Input: part model. Units: mm. Frame: model coordinates. Face numbers are marked on the shaded views. A direction names the side the tool comes from. Give positions to 0.01 mm unless a question says otherwise; leave off trailing zeros. Loops run counter-clockwise (first coordinate to the right, second up) from the corner with the lowest first, then second, coordinate; pieces in that order, holes last. Notation, with made-up numbers: M 54.5,-30 L 98.5,-30 A28 cw 98.5,1 Z; hole C 54,9.5 d7. An arc over 180 degrees is marked long. One line per item, written item: value. Start each with the question number.
(1) Ray query, line 1 along X through (y, z) = (1.4, 15); line 2 along Y through (x, z) = (0.75, 2); line 3 along Z through (x, y) = (-5, -0.2). Return the intervals inside material, ascending. Write a range as from..to.
(2) Section D-D on x = -1.25. Output: boundary loops of the cut face in (y, z), plus the area to 3 significant figures.
(3) Pin query (flat end, axial travel): P1, Ø0.5, axis at y = 1.5, z = 14.5, coming from the +X side; P2, Ø0.5, axis at x = -5.5, z = 7.5, coming from the -Y side; P3, Ø2, axis at y = -0.5, z = -1.5, coming from the -X side. Return the tip coordinate at first contact, or that it passes through.
(4) Access query for the marked faces 1 and 2. Directions: +Z, -Z, +X, -X, +Y, -Y. A direction counts if a zero-diameter tool reaches every point of the face in a straight line with its end or side. Return the directions, or none.
(5) Section C-C on x = 5.25. Output: boundary loops of the cut face in (y, z).
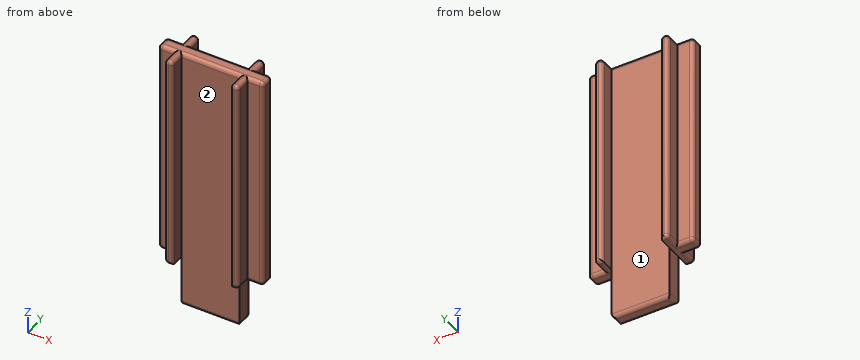
```python
from build123d import *

# Parameters (mm, degrees)
AUFSATZ_LINEAR_AUSTRAGEN1_DEPTH = 28
SKIZZE2_W                       = 7.5
SKIZZE2_H                       = 1.8
AUFSATZ_LINEAR_AUSTRAGEN2_DEPTH = 6.63
VERRUNDUNG1_R                   = 0.5


with BuildPart() as part:
    # Skizze1 → Aufsatz-Linear austragen1 (new body)
    with BuildSketch(Plane.XY):
        Polygon((-4.75, 0.9), (-6.8, 0.9), (-6.8, -0.9), (-4.75, -0.9), (-4.75, -2.9), (-3.75, -2.9), (-3.75, -0.9), (3.75, -0.9), (3.75, -2.9), (4.75, -2.9), (4.75, -0.9), (6.8, -0.9), (6.8, 0.9), (4.75, 0.9), (4.75, 2.9), (3.75, 2.9), (3.75, 0.9), (-3.75, 0.9), (-3.75, 2.9), (-4.75, 2.9), align=None)
    extrude(amount=AUFSATZ_LINEAR_AUSTRAGEN1_DEPTH)

    # Skizze2 → Aufsatz-Linear austragen2 (add)
    with BuildSketch(Plane(origin=(0, 0, 0), x_dir=(-1, 0, 0), z_dir=(0, 0, -1))):
        Rectangle(SKIZZE2_W, SKIZZE2_H)
    extrude(amount=AUFSATZ_LINEAR_AUSTRAGEN2_DEPTH)

    # Verrundung1
    verrundung1_edges = [part.edges().sort_by_distance(p)[0] for p in [
        (-4.75, -1.9, 28),
        (-4.25, -2.9, 28),
        (-5.775, 0.9, 0),
        (-4.75, 1.9, 0),
        (-4.25, 2.9, 0),
        (-3.75, -1.9, 28),
        (4.25, 2.9, 0),
        (4.75, 1.9, 0),
        (5.775, 0.9, 0),
        (6.8, 0, 0),
        (5.775, -0.9, 0),
        (4.75, -1.9, 0),
        (4.25, -2.9, 0),
        (0, -0.9, 28),
        (-4.25, -2.9, 0),
        (-4.75, -1.9, 0),
        (-5.775, -0.9, 0),
        (-6.8, 0, 0),
        (3.75, -1.9, 28),
        (4.25, -2.9, 28),
        (-6.8, 0.9, 14),
        (-4.75, 2.9, 14),
        (-3.75, 2.9, 14),
        (3.75, 2.9, 14),
        (4.75, 2.9, 14),
        (6.8, 0.9, 14),
        (6.8, -0.9, 14),
        (4.75, -2.9, 14),
        (3.75, -2.9, 14),
        (-3.75, -2.9, 14),
        (-4.75, -2.9, 14),
        (-6.8, -0.9, 14),
        (4.75, -1.9, 28),
        (5.775, -0.9, 28),
        (6.8, 0, 28),
        (5.775, 0.9, 28),
        (-6.8, 0, 28),
        (4.75, 1.9, 28),
        (4.25, 2.9, 28),
        (3.75, 0, -6.63),
        (0, -0.9, -6.63),
        (-3.75, 0, -6.63),
        (0, 0.9, -6.63),
        (3.75, 1.9, 28),
        (0, 0.9, 28),
        (-3.75, 1.9, 28),
        (-4.25, 2.9, 28),
        (-4.75, 1.9, 28),
        (-5.775, 0.9, 28),
        (-5.775, -0.9, 28),
    ]]
    fillet(verrundung1_edges, radius=VERRUNDUNG1_R - 0.0001)  # a hair under: the kernel refuses the full size


solid = part.part
```
Output values:
1. line 1: x = -4.75..-3.75, 3.75..4.75
1. line 2: y = -0.9..0.9
1. line 3: z = 0..28
2. outline: M -0.9,-6.13 A0.5 ccw -0.4,-6.63 L 0.4,-6.63 A0.5 ccw 0.9,-6.13 L 0.9,27.5 A0.5 ccw 0.4,28 L -0.4,28 A0.5 ccw -0.9,27.5 Z
2. area: 62.1 mm²
3. P1: stops at x = 4.75
3. P2: stops at y = -0.9
3. P3: stops at x = -3.75
4. face 1: +Z, -Z, +Y
4. face 2: +Z, -Z, -Y
5. outline: M -0.9,0.5 A0.5 ccw -0.4,0 L 0.4,0 A0.5 ccw 0.9,0.5 L 0.9,27.5 A0.5 ccw 0.4,28 L -0.4,28 A0.5 ccw -0.9,27.5 Z
